Autodesk Inventor part; units mm, degrees
ref_plane "YZ Plane" through (0, 0, 0) normal (1, 0, 0) x (0, 1, 0)
ref_plane "XZ Plane" through (0, 0, 0) normal (0, 1, 0) x (-1, 0, 0)
ref_plane "XY Plane" through (0, 0, 0) normal (0, 0, 1) x (1, 0, 0)
sketch "スケッチ1" plane through (0, 0, 0) normal (0, 0, 1) x (1, 0, 0)
  line L0 (-1.9, 5) -> (0, 5)
  line L1 (1.9, 5) -> (1.9, 3)
  line L2 (1.9, 3) -> (-1.9, 3)
  line L3 (-1.9, 3) -> (-1.9, 5)
  line L4 (-1, 3) -> (0, 3)
  line L5 (1, 3) -> (1, -2)
  line L6 (1, -2) -> (0, -2)
  line L7 (-1, -2) -> (-1, 3)
  line L8 (0, 5) -> (0, -2)
  line L9 (0, 5) -> (1.9, 5)
  line L10 (0, 3) -> (1, 3)
  line L11 (0, -2) -> (-1, -2)
  point P0 (0, 0)
  dimension "d0" = 2
  dimension "d1" = 1
  dimension "d2" = 5
  dimension "d3" = 3.8
  dimension "d4" = 1.9
  dimension "d5" = 2
revolve "回転1" add sketch "スケッチ1" angle 360 about axis through (0, 5, 0) along (0, -1, 0) contours L0 L8 L2 L3 | L8 L11 L7 L2
thread "ねじ1"
sketch "スケッチ2" plane through (0, 5, 0) normal (0, 1, 0) x (1, 0, 0)
  line L0 (0, 0.866) -> (0.75, 0.433)
  line L1 (0.75, 0.433) -> (0.75, -0.433)
  line L2 (0.75, -0.433) -> (0, -0.866)
  line L3 (0, -0.866) -> (-0.75, -0.433)
  line L4 (-0.75, -0.433) -> (-0.75, 0.433)
  line L5 (-0.75, 0.433) -> (0, 0.866)
  point P0 (0, 0)
  dimension "d9" = 1.5
extrude "押し出し1" cut sketch "スケッチ2" against normal blind 2
chamfer "面取り1" distance 0.1 angle 45 2 edges at (1.9, 5, 0) (1.9, 3, 0)
chamfer "面取り2" distance 0.2 angle 45 6 edges at (0.375, 5, 0.6495) (-0.375, 5, 0.6495) (-0.75, 5, 0) (-0.375, 5, -0.6495) (0.375, 5, -0.6495) (0.75, 5, 0)
properties part number "M2_5mm"
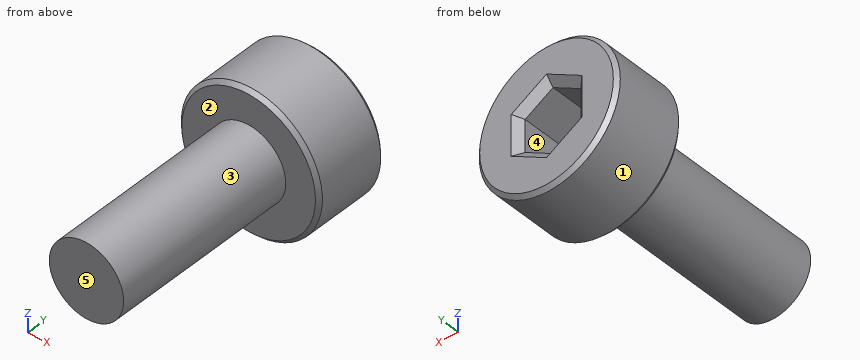
The model under review builds one solid part; all positions refer to its coordinate system, in mm. Face numbers are marked on the shaded views. A direction names the side the tool comes from. Round coordinates to 2 decimals unless told otherwise and drop trailing zeros. Write each loop counter-clockwise with the first axis right and the second up, starting at its lowest first coordinate (ties: lowest second). Pieces come first, ordered by that corner, then holes. Notation, with made-up numbers: (25, -27) - (54, -27) arc R26 cw to (54, -4) - close; hole circle Ø1 at (20.25, 73). An arc over 180 degrees is marked (long way). Answer as CSV lines item,"result". Start each with the question number.
(1) Draft analysis for pull direction X (two halves, no side actions). For the marked faces 3, 4 and 5, state which applies: pulls with the +X half, pulls with the -X half, needs draft (parallel to the pull), parting line crosses it, or undercut.
(2) For the marked faces 1 and 2, list the 3-axis set-ups (+Z, -Z, +X, -X, +Y, -Y) from which the entire face can be reached by the end or side of a thin tool; tool diameter is ignored.
(3) For pin 1 Ø1.5 at (x, z) = (1, 1.5) entering from -Y, flat-tipped, find the tip position at first contact; note if it passes through.
(4) We need section A-A on y = 3.25. State the section outline as (x, z) points.
(5) To check wall thickness, follow line 1 (Y direction, x = 0.3, z = 0.1); line 2 (X direction, y = 1.25, z = -0.5); line 3 (X direction, y = 4, z = -0.05). State the ranges of each line that lie inside material, in increasing order.
(6) We need section C-C on y = -1. State the section outline as (x, z) points, plus the area to 3 significant figures.
(7) We need section B-B on z = 0. State the section outline as (x, y) points, plus the area to 3 significant figures.
Worked answers:
1,face 3,"parting line crosses it"
1,face 4,"undercut"
1,face 5,"needs draft"
2,face 1,"+Y, -Y"
2,face 2,"-Y"
3,pin 1,"y = 3"
4,outline,"circle Ø3.8 at (0, 0); hole (-0.75, -0.43) - (0, -0.87) - (0.75, -0.43) - (0.75, 0.43) - (0, 0.87) - (-0.75, 0.43) - close"
5,line 1,"-2 to 3"
5,line 2,"-0.87 to 0.87"
5,line 3,"-1.9 to -0.75, 0.75 to 1.9"
6,outline,"circle Ø2 at (0, 0)"
6,area,"3.14 mm²"
7,outline,"(-1.9, 3.1) - (-1.8, 3) - (-1, 3) - (-1, -2) - (1, -2) - (1, 3) - (1.8, 3) - (1.9, 3.1) - (1.9, 4.9) - (1.8, 5) - (0.95, 5) - (0.75, 4.8) - (0.75, 3) - (-0.75, 3) - (-0.75, 4.8) - (-0.95, 5) - (-1.8, 5) - (-1.9, 4.9) - close"
7,area,"14.5 mm²"
